Verification items for the finished model (mm, model axes). A direction names the side the tool comes from. Coordinates: 2 decimals unless noted, no trailing zeros. Order: outer loops, then holes, each group sorted by start corner. A loop starts at its lowest first (then second) coordinate and runs counter-clockwise, first axis right, second up. Notation, with made-up numbers: (-31, 46.5) -> (-27, 46.5) arc R14 ccw to (-27, 63.5) -> close; hole circle Ø8 at (27, 27.25). An arc over 180 degrees is marked (long way). Answer as CSV lines item,"result".
```python
from build123d import *

# Parameters (mm, degrees)
BOSS_EXTRUDE1_DEPTH     = 127
SKETCH2_R               = 2.049999964
SKETCH2_W               = 19.05
SKETCH2_H               = 8.89
CUT_EXTRUDE1_DEPTH      = 25.48749992
FILLET1_R               = 12.7
BOSS_EXTRUDE2_REACH     = 18.672
SKETCH4_W               = 1.891908828
SKETCH4_H               = 8.89
BOSS_EXTRUDE3_DEPTH     = 12.7
SKETCH6_W               = 15.875
SKETCH6_H               = 12.7
CUT_EXTRUDE2_DEPTH      = 25.48749992
BOSS_EXTRUDE4_DEPTH     = 127
SKETCH8_R               = 2.200000045
SKETCH8_W               = 17.833904447
SKETCH8_H               = 8.89
SKETCH8_W_2             = 15.875
SKETCH8_H_2             = 12.7
CUT_EXTRUDE3_DEPTH      = 23.89999992
CUT_EXTRUDE3_DEPTH_BACK = 5.1275
SKETCH9_W               = 4.918962954
SKETCH9_H               = 8.89
CUT_EXTRUDE4_DEPTH      = 22.500442069
FILLET2_R               = 1
FILLET3_R               = 1
BOSS_EXTRUDE5_DEPTH     = 114.3
BOSS_EXTRUDE6_DEPTH     = 12.7
CUT_EXTRUDE5_DEPTH      = 23.89999992
FILLET4_R               = 1


with BuildPart() as part:
    # Sketch1 → Boss-Extrude1 (new body)
    with BuildSketch(Plane(origin=(0, 0, 0), x_dir=(1, 0, 0), z_dir=(0, 1, 0))):
        with BuildLine():
            Line((0, 0), (-35.56, 0))
            ThreePointArc((-35.56, 0), (-39.585438943, -0.892418328), (-42.856573321, -3.402448018))
            Line((-42.856573321, -3.402448018), (-59.216961931, -22.89999992))
            Line((-59.216961931, -22.89999992), (-60.433057484, -21.87957459))
            Line((-60.433057484, -21.87957459), (-44.072668874, -2.382022687))
            ThreePointArc((-44.072668874, -2.382022687), (-40.256345434, 0.546345283), (-35.56, 1.5875))
            Line((-35.56, 1.5875), (0, 1.5875))
            Line((0, 1.5875), (0, 0))
        make_face()
    extrude(amount=BOSS_EXTRUDE1_DEPTH)

    # Sketch2 → Cut-Extrude1 (cut, through all)
    with BuildSketch(Plane(origin=(0, 0, -1.5875), x_dir=(-1, 0, 0), z_dir=(0, 0, -1))):
        with Locations((8.399999964, 88.9)):
            Circle(SKETCH2_R)
        with Locations((8.399999964, 60.116067728)):
            Circle(SKETCH2_R)
        with Locations((39.514999964, 88.9)):
            Rectangle(SKETCH2_W, SKETCH2_H)
        with Locations((39.514999964, 60.116067728)):
            Rectangle(SKETCH2_W, SKETCH2_H)
    extrude(amount=-CUT_EXTRUDE1_DEPTH, mode=Mode.SUBTRACT)

    # Fillet1
    fillet1_edges = [part.edges().sort_by_distance(p)[0] for p in [
        (0, 0, -0.79375),
        (-59.825009707, 127, 22.389787255),
        (0, 127, -0.79375),
        (-59.825009707, 0, 22.389787255),
    ]]
    fillet(fillet1_edges, radius=FILLET1_R)

    # Boss-Extrude2: up to this face of the body (flat: up to its plane)
    boss_extrude2_end = Plane(part.part.faces().sort_by_distance((-49.039999964, 88.9, 9.536713147))[0])
    # Sketch4 → Boss-Extrude2 (add, up to the picked face)
    with BuildSketch(Plane(origin=(-23.473890996, 0, -19.696933277), x_dir=(0.64278761, 0, -0.766044443), z_dir=(0.766044443, 0, 0.64278761)), mode=Mode.PRIVATE) as boss_extrude2_sk1:
        with Locations((-38.827850468, 88.9)):
            Rectangle(SKETCH4_W, SKETCH4_H)
    boss_extrude2_tool1 = split(extrude(boss_extrude2_sk1.sketch, amount=-BOSS_EXTRUDE2_REACH, mode=Mode.PRIVATE), bisect_by=boss_extrude2_end, keep=Keep.BOTH, mode=Mode.PRIVATE)
    add(boss_extrude2_tool1.solids().sort_by_distance((-48.431952, 88.9, 10.046926))[0])
    # Sketch4 → Boss-Extrude2 (add, up to the picked face)
    with BuildSketch(Plane(origin=(-23.473890996, 0, -19.696933277), x_dir=(0.64278761, 0, -0.766044443), z_dir=(0.766044443, 0, 0.64278761)), mode=Mode.PRIVATE) as boss_extrude2_sk2:
        with Locations((-38.827850468, 60.116067728)):
            Rectangle(SKETCH4_W, SKETCH4_H)
    boss_extrude2_tool2 = split(extrude(boss_extrude2_sk2.sketch, amount=-BOSS_EXTRUDE2_REACH, mode=Mode.PRIVATE), bisect_by=boss_extrude2_end, keep=Keep.BOTH, mode=Mode.PRIVATE)
    add(boss_extrude2_tool2.solids().sort_by_distance((-48.431952, 60.116068, 10.046926))[0])

    # Sketch5 → Boss-Extrude3 (add)
    with BuildSketch(Plane.XZ):
        with BuildLine():
            Line((-44.072668874, 2.382022687), (-60.433057484, 21.87957459))
            Line((-60.433057484, 21.87957459), (-59.216961931, 22.89999992))
            Line((-59.216961931, 22.89999992), (0, 22.89999992))
            Line((0, 22.89999992), (0, -1.5875))
            Line((0, -1.5875), (-35.56, -1.5875))
            ThreePointArc((-35.56, -1.5875), (-40.256345434, -0.546345283), (-44.072668874, 2.382022687))
        make_face()
    extrude(amount=-BOSS_EXTRUDE3_DEPTH)

    # Sketch6 → Cut-Extrude2 (cut, through all)
    with BuildSketch(Plane(origin=(0, 0, -1.5875), x_dir=(-1, 0, 0), z_dir=(0, 0, -1))):
        with Locations((7.9375, 6.35)):
            Rectangle(SKETCH6_W, SKETCH6_H)
    extrude(amount=-CUT_EXTRUDE2_DEPTH, mode=Mode.SUBTRACT)

    # Sketch7 → Boss-Extrude4 (add)
    with BuildSketch(Plane.XZ):
        with BuildLine():
            Line((-59.216961931, 22.89999992), (-64.605030517, 22.89999992))
            Line((-64.605030517, 22.89999992), (-46.01842176, 0.749342159))
            ThreePointArc((-46.01842176, 0.749342159), (-41.329795818, -2.848367063), (-35.56, -4.1275))
            Line((-35.56, -4.1275), (0, -4.1275))
            Line((0, -4.1275), (0, -1.5875))
            Line((0, -1.5875), (-15.875, -1.5875))
            Line((-15.875, -1.5875), (-35.56, -1.5875))
            ThreePointArc((-35.56, -1.5875), (-40.256345434, -0.546345283), (-44.072668874, 2.382022687))
            Line((-44.072668874, 2.382022687), (-52.269654841, 12.150810162))
            Line((-52.269654841, 12.150810162), (-51.053559288, 13.171235492))
            Line((-51.053559288, 13.171235492), (-59.216961931, 22.89999992))
        make_face()
    extrude(amount=-BOSS_EXTRUDE4_DEPTH)

    # Sketch8 → Cut-Extrude3 (cut, two sides)
    with BuildSketch(Plane.XY) as cut_extrude3_sk:
        with Locations((-8.399999964, 88.9)):
            Circle(SKETCH8_R)
        with Locations((-8.399999964, 60.116067728)):
            Circle(SKETCH8_R)
        with BuildLine():
            Line((-12.7, 127), (0, 127))
            Line((0, 127), (0, 114.3))
            ThreePointArc((0, 114.3), (-3.719743879, 123.280256121), (-12.7, 127))
        make_face()
        with Locations((-38.906952188, 88.9)):
            Rectangle(SKETCH8_W, SKETCH8_H)
        with Locations((-38.906952188, 60.116067728)):
            Rectangle(SKETCH8_W, SKETCH8_H)
        with Locations((-7.9375, 6.35)):
            Rectangle(SKETCH8_W_2, SKETCH8_H_2)
    extrude(amount=CUT_EXTRUDE3_DEPTH, mode=Mode.SUBTRACT)
    extrude(cut_extrude3_sk.sketch, amount=-CUT_EXTRUDE3_DEPTH_BACK, mode=Mode.SUBTRACT)

    # Sketch9 → Cut-Extrude4 (cut, through all)
    with BuildSketch(Plane(origin=(-23.473890996, 0, -19.696933277), x_dir=(0.64278761, 0, -0.766044443), z_dir=(0.766044443, 0, 0.64278761))):
        with Locations((-35.422414577, 88.9)):
            Rectangle(SKETCH9_W, SKETCH9_H)
        with Locations((-35.422414577, 60.116067728)):
            Rectangle(SKETCH9_W, SKETCH9_H)
    extrude(amount=-CUT_EXTRUDE4_DEPTH, mode=Mode.SUBTRACT)

    # Fillet2
    fillet2_edges = [part.edges().sort_by_distance(p)[0] for p in [
        (0, 12.7, -2.06375),
        (-15.875, 12.7, 11.44999996),
        (-15.875, 0, 9.38624996),
        (-64.605030517, 63.5, 22.89999992),
    ]]
    fillet(fillet2_edges, radius=FILLET2_R)

    # Fillet3
    fillet3_edges = [part.edges().sort_by_distance(p)[0] for p in [
        (-15.875, 12.7, -2.06375),
    ]]
    fillet(fillet3_edges, radius=FILLET3_R)

    # Sketch10 → Boss-Extrude5 (add)
    with BuildSketch(Plane(origin=(0, 12.7, 0), x_dir=(1, 0, 0), z_dir=(0, 1, 0))):
        Polygon((-59.216961931, -22.89999992), (-54.136961931, -22.89999992), (-54.136961931, -16.84589167), align=None)
    extrude(amount=BOSS_EXTRUDE5_DEPTH)

    # Sketch11 → Boss-Extrude6 (add)
    with BuildSketch(Plane(origin=(0, 114.3, 0), x_dir=(1, 0, 0), z_dir=(0, 1, 0))):
        with BuildLine():
            Line((-54.136961931, -22.89999992), (-54.136961931, -16.84589167))
            Line((-54.136961931, -16.84589167), (-42.856573321, -3.402448018))
            ThreePointArc((-42.856573321, -3.402448018), (-39.585438943, -0.892418328), (-35.56, 0))
            Line((-35.56, 0), (0, 0))
            Line((0, 0), (0, -22.89999992))
            Line((0, -22.89999992), (-54.136961931, -22.89999992))
        make_face()
    extrude(amount=BOSS_EXTRUDE6_DEPTH)

    # Sketch12 → Cut-Extrude5 (cut, through all)
    with BuildSketch(Plane(origin=(0, 0, 0), x_dir=(-1, 0, 0), z_dir=(0, 0, -1))):
        with BuildLine():
            Line((12.7, 127), (0, 127))
            Line((0, 127), (0, 114.3))
            ThreePointArc((0, 114.3), (3.719743879, 123.280256121), (12.7, 127))
        make_face()
    extrude(amount=-CUT_EXTRUDE5_DEPTH, mode=Mode.SUBTRACT)

    # Fillet4
    fillet4_edges = [part.edges().sort_by_distance(p)[0] for p in [
        (0, 114.3, 11.44999996),
    ]]
    fillet(fillet4_edges, radius=FILLET4_R)


solid = part.part
```
Item 1: Thickness scan on line 1 (Y direction, x = -32, z = -3) (3 decimals); line 2 (Y direction, x = -42.5, z = 4.5); line 3 (Y direction, x = -8.4, z = -1.25). Record the ranges inside material, lowest first.
Answer list:
line 1,"0 to 55.671, 64.561 to 84.455, 93.345 to 127"
line 2,"0 to 12.7, 114.3 to 127"
line 3,"12.7 to 57.92, 62.32 to 86.7, 91.1 to 126.25"
Item 2: Section check C-C, the plane z = 5.5. Record the boundary of the cut face in (x, y) (3 decimals), plus the area to 3 significant figures.
Answer list:
outline,"(-50.005, 0) -> (-16.875, 0) arc R1 ccw to (-15.875, 1) -> (-15.875, 11.7) arc R1 ccw to (-16.875, 12.7) -> (-44.617, 12.7) -> (-44.617, 55.671) -> (-50.005, 55.671) -> close; (-50.005, 64.561) -> (-44.617, 64.561) -> (-44.617, 84.455) -> (-50.005, 84.455) -> close; (-50.005, 93.345) -> (-44.617, 93.345) -> (-44.617, 114.3) -> (-1.043, 114.3) arc R1 ccw to (-0.046, 115.385) arc R12.7 ccw to (-12.7, 127) -> (-50.005, 127) -> close"
area,"1,480 mm2"
Item 3: Release check for a two-part mould opening along Y. For faces 5 (the flat face through (0, 63, -2)), 6 (the flat face through (-8, 12.7, -2)), 7 (the flat face through (-40.3, 84.455, 1)) record: +Y half, -Y half, draft (parallel to the pull), parting line (faces both ways), or undercut.
Answer list:
face 5,"draft"
face 6,"-Y half"
face 7,"undercut"
Item 4: Section check B-B, the plane y = 88.9. Record the boundary of the cut face in (x, z), plus the area to 3 significant figures.
Answer list:
outline,"(-63.23, 21.26) -> (-50.99, 6.67) -> (-47.82, 9.32) -> (-54.14, 16.85) -> (-54.14, 22.9) -> (-62.46, 22.9) arc R1 ccw to start; (-29.99, -4.13) -> (-10.6, -4.13) -> (-10.6, 0) -> (-29.99, 0) -> close; (-6.2, -4.13) -> (0, -4.13) -> (0, 0) -> (-6.2, 0) -> close"
area,"200 mm2"
Item 5: Tool access check on faces 1 (the flat face through (-15.875, 6, 9)), 2 (the flat face through (-29.99, 60, -2)), 3 (the flat face through (-18, 63, 0)), 4 (the flat face through (-49.4, 88.8, 8)). Record the directions out of +Z, -Z, +X, -X, +Y, -Y that give a thin tool (end or side, any length) a straight path to the whole face; none if there is none.
Answer list:
face 1,"+Z, -Z, +X, -Y"
face 2,"+Z, -Z, -X"
face 3,"+Z, +X"
face 4,"-Z, +X"
Item 6: Section check A-A, the plane x = -32. Record the boundary of the cut face in (y, z) (1 decimal), plus the area to 3 significant figures.
Answer list:
outline,"(0, -4.1) -> (55.7, -4.1) -> (55.7, 0) -> (12.7, 0) -> (12.7, 22.9) -> (0, 22.9) -> close; (64.6, -4.1) -> (84.5, -4.1) -> (84.5, 0) -> (64.6, 0) -> close; (93.3, -4.1) -> (127, -4.1) -> (127, 22.9) -> (114.3, 22.9) -> (114.3, 0) -> (93.3, 0) -> close"
area,"1,030 mm2"
Item 7: Depth check by flat-ended pin: pin 1 Ø2 at (x, z) = (-6.5, -1.5) entering from -Y; pin 2 Ø4 at (x, y) = (-13.5, 14.5) entering from +Z; pin 3 Ø4 at (y, z) = (25.5, 11) entering from -X. Enter the tip coordinate at first touch or a pass-through.
Answer list:
pin 1,"y = 12.7"
pin 2,"z = 0"
pin 3,"x = -56.3"
